Geometry: final body of the model. Coordinates: model frame, mm. A direction names the side the tool comes from. Coordinates: 2 decimals unless noted, no trailing zeros. Loops run counter-clockwise (first coordinate to the right, second up) from the corner with the lowest first, then second, coordinate; pieces in that order, holes last. Notation, with made-up numbers: (19, 86.25) -> (64, 86.25) arc R31 cw to (64, 119.25) -> close; hole circle Ø7 at (35.25, 45). An arc over 180 degrees is marked (long way). One line per item, written item: value. Start each with the question number.
Item 1: Set-up query: faces 1 (the flat face through (0, 26, -15)), 2 (the cylindrical face through (22.715, 48.958, -3.301)), 3 (the flat face through (7, 46, -2)). Return all of +Z, -Z, +X, -X, +Y, -Y with unobstructed straight access to the full face (end or side cutting, diameter ignored); none if empty.
Item 2: Section query B-B on z = -20.5. Return loops of the section in (x, y) (3 decimals), then the cut area to 4 significant figures.
Item 3: Section query D-D on z = -9. Return loops of the section in (x, y) (3 decimals), then the cut area to 3 significant figures.
Item 4: Mould query, pull axis Y, two halves, no side actions, for faces 4 (the flat face through (13, 49, -3)), 5 (the flat face through (3, 29, -15)), 6 (the cylindrical face through (25.43, 51.4, -14.71)), 7 (the flat face through (13, 0, -15)). Classes: +Y half, -Y half, draft (parallel to the pull), parting line (faces both ways), or undercut.
Item 5: Section query A-A on y = 36. Return loops of the section in (x, z), then the cut area to 3 significant figures.
Item 6: Section query C-C on x = 7.9. Return loops of the section in (y, z) (3 decimals).
Item 7: Ray query, probe 1 along Y at (x, z) = (18.1, -21) (3 decimals); probe 2 along X at (y, z) = (40.5, -3.5); probe 3 along Y at (x, z) = (16.75, -18.25). Return the intervals inside material, ascending. Write a range as from..to.
Autodesk Inventor part; units mm, degrees
ref_plane "YZ Plane" through (0, 0, 0) normal (1, 0, 0) x (0, 1, 0)
ref_plane "XZ Plane" through (0, 0, 0) normal (0, 1, 0) x (-1, 0, 0)
ref_plane "XY Plane" through (0, 0, 0) normal (0, 0, 1) x (1, 0, 0)
sketch "Sketch6" plane through (0, 0, 0) normal (0, 0, 1) x (1, 0, 0)
  line L0 (2, 0) -> (24, 0)
  line L1 (24, 52) -> (2, 52)
  line L2 (0, 50) -> (0, 2)
  line L3 (3, 6) -> (23, 6)
  line L4 (23, 6) -> (23, 46)
  line L5 (13, 6) -> (13, 46) construction
  line L6 (16, 46) -> (16, 48)
  line L7 (10, 48) -> (10, 46)
  line L8 (23, 46) -> (16, 46)
  line L9 (10, 46) -> (3, 46)
  arc A0 (2, 52) -> (0, 50) centre (2, 50) ccw
  arc A1 (26, 50) -> (24, 52) centre (24, 50) ccw
  arc A2 (24, 0) -> (26, 2) centre (24, 2) ccw
  arc A3 (0, 2) -> (2, 0) centre (2, 2) ccw
  line L10 (3, 26) -> (23, 26) construction
  line L11 (26, 2) -> (26, 50)
  line L12 (3, 46) -> (3, 6)
  line L13 (10, 48) -> (16, 48)
  point P0 (0, 0)
  dimension "d122" = 52
  dimension "d126" = 6
  dimension "d127" = 6
  dimension "d131" = 3
  dimension "d132" = 2
  dimension "d159" = 13
  dimension "d162" = 10
  dimension "d163" = 10
  dimension "d164" = 3
  dimension "d165" = 3
  dimension "d166" = 20
  dimension "d167" = 40
extrude "Extrusion3" add sketch "Sketch6" against normal blind 29.833
sketch "Sketch7" plane through (0, 0, 0) normal (0, 0, 1) x (1, 0, 0)
  point P0 (0, 0)
sketch "Sketch8" plane through (0, 0, 0) normal (0, 0, 1) x (1, 0, 0)
  circle A0 centre (7.9, 49.9) radius 1.095
  circle A1 centre (18.1, 49.9) radius 1.095
  line L0 (3, 46) -> (10, 46)
  line L1 (16, 46) -> (23, 46)
  line L2 (10, 48) -> (16, 48)
  line L3 (13, 48) -> (13, 6) construction
  line L4 (3, 6) -> (23, 6)
  line L5 (5, 6) -> (5, 46)
  line L6 (5, 26) -> (23, 26) construction
  line L7 (23, 46) -> (23, 6)
  circle A2 centre (7.9, 2.1) radius 1.095
  circle A3 centre (18.1, 2.1) radius 1.095
  point P0 (0, 0)
  dimension "d149" = 2.19
  dimension "d150" = 2.19
  dimension "d151" = 3.9
  dimension "d152" = 3.9
  dimension "d153" = 5.1
  dimension "d154" = 5.1
extrude "Extrusion4" cut sketch "Sketch8" against normal blind 33.25
sketch "Sketch9" plane through (2, 52, 0) normal (0, 1, 0) x (1, 0, 0)
  line L0 (1, 3) -> (21, 3)
  line L1 (21, 3) -> (21, 11)
  line L2 (21, 11) -> (1, 11)
  line L3 (1, 11) -> (1, 3)
  line L4 (22, 0) -> (0, 0)
  line L5 (0, 0) -> (0, 29.833)
  point P0 (-2, 0)
  dimension "d168" = 20
  dimension "d169" = 8
  dimension "d171" = 3
  dimension "d172" = 1
extrude "Extrusion5" cut sketch "Sketch9" against normal blind 6
fillet "Fillet1" radius 1 1 edges at (23, 49, -11)
fillet "Fillet2" radius 1 3 edges at (23, 49, -3) (3, 49, -11) (3, 49, -3)
properties part number "NewServoMount"
Reply:
1. face 1: +Z, -Z, -X, +Y, -Y
1. face 2: +Y
1. face 3: +Z, -Z
2. outline: (0, 2) arc R2 ccw to (2, 0) -> (24, 0) arc R2 ccw to (26, 2) -> (26, 50) arc R2 ccw to (24, 52) -> (2, 52) arc R2 ccw to (0, 50) -> close; hole (3, 6) -> (23, 6) -> (23, 46) -> (16, 46) -> (16, 48) -> (10, 48) -> (10, 46) -> (3, 46) -> close; hole circle Ø2.19 at (7.9, 2.1); hole circle Ø2.19 at (7.9, 49.9); hole circle Ø2.19 at (18.1, 2.1); hole circle Ø2.19 at (18.1, 49.9)
2. area: 521.5 mm²
3. outline: (0, 2) arc R2 ccw to (2, 0) -> (24, 0) arc R2 ccw to (26, 2) -> (26, 50) arc R2 ccw to (24, 52) -> (23, 52) -> (23, 6) -> (3, 6) -> (3, 52) -> (2, 52) arc R2 ccw to (0, 50) -> close; hole circle Ø2.19 at (7.9, 2.1); hole circle Ø2.19 at (18.1, 2.1)
3. area: 421 mm²
4. face 4: draft
4. face 5: undercut
4. face 6: +Y half
4. face 7: -Y half
5. outline: (0, -29.83) -> (3, -29.83) -> (3, 0) -> (0, 0) -> close; (23, -29.83) -> (26, -29.83) -> (26, 0) -> (23, 0) -> close
5. area: 179 mm²
6. outline: (0, -29.833) -> (1.005, -29.833) -> (1.005, 0) -> (0, 0) -> close; (3.195, -29.833) -> (6, -29.833) -> (6, 0) -> (3.195, 0) -> close; (46, -29.833) -> (48.805, -29.833) -> (48.805, -11) -> (46, -11) -> close; (46, -3) -> (48.805, -3) -> (48.805, 0) -> (46, 0) -> close; (50.995, -29.833) -> (52, -29.833) -> (52, -11) -> (50.995, -11) -> close; (50.995, -3) -> (52, -3) -> (52, 0) -> (50.995, 0) -> close
7. probe 1: y = 0..1.005, 3.195..6, 46..48.805, 50.995..52
7. probe 2: x = 0..3, 23..26
7. probe 3: y = 0..6, 46..52
